from build123d import *

# Parameters (mm, degrees)
SKETCH1_R                 = 12.1666
SKETCH1_R_2               = 10.5791
BOSS_EXTRUDE1_DEPTH       = 19.05
SKETCH2_W                 = 25.4
SKETCH2_H                 = 28.575
BOSS_EXTRUDE2_DEPTH       = 3.175
SKETCH3_R                 = 6.35
CUT_EXTRUDE1_DEPTH        = 23.225
SKETCH8_R                 = 10.5791
SKETCH8_R_2               = 6.35
BOSS_EXTRUDE4_DEPTH       = 0.127
SKETCH9_R                 = 10.5791
SKETCH9_R_2               = 3.96875
BOSS_EXTRUDE5_DEPTH       = 3.175
F_2_56_TAPPED_HOLE1_D     = 1.778
F_2_56_TAPPED_HOLE1_DEPTH = 5.588
F_2_56_TAPPED_HOLE1_TIP   = 0.53416509
SKETCH6_W                 = 15.875
SKETCH6_H                 = 37.082262956
CUT_EXTRUDE2_DEPTH        = 1.5875


with BuildPart() as part:
    # Sketch1 → Boss-Extrude1 (new body)
    with BuildSketch(Plane(origin=(0, 0, 0), x_dir=(1, 0, 0), z_dir=(0, 1, 0))):
        Circle(SKETCH1_R)
        Circle(SKETCH1_R_2, mode=Mode.SUBTRACT)
    extrude(amount=BOSS_EXTRUDE1_DEPTH)

    # Sketch2 → Boss-Extrude2 (add)
    with BuildSketch(Plane.XZ):
        with Locations((0, 2.1209)):
            Rectangle(SKETCH2_W, SKETCH2_H)
    extrude(amount=BOSS_EXTRUDE2_DEPTH)

    # Sketch3 → Cut-Extrude1 (cut, through all)
    with BuildSketch(Plane.XZ.offset(3.175)):
        Circle(SKETCH3_R)
    extrude(amount=-CUT_EXTRUDE1_DEPTH, mode=Mode.SUBTRACT)

    # Sketch8 → Boss-Extrude4 (add)
    with BuildSketch(Plane(origin=(0, 0, 0), x_dir=(1, 0, 0), z_dir=(0, 1, 0))):
        Circle(SKETCH8_R)
        Circle(SKETCH8_R_2, mode=Mode.SUBTRACT)
    extrude(amount=BOSS_EXTRUDE4_DEPTH)

    # Sketch9 → Boss-Extrude5 (add)
    with BuildSketch(Plane(origin=(0, 0.127, 0), x_dir=(1, 0, 0), z_dir=(0, 1, 0))):
        Circle(SKETCH9_R)
        Circle(SKETCH9_R_2, mode=Mode.SUBTRACT)
    extrude(amount=BOSS_EXTRUDE5_DEPTH)

    # #2-56 Tapped Hole1
    with Locations(Plane(origin=(0, -3.175, 0), x_dir=(-1, 0, 0), z_dir=(0, -1, 0))):
        with Locations((10.531523735, -12.441379328), (10.531523735, 0.058620672), (-10.468476265, -12.441379328), (-10.468476265, 0.058620672)):
            Hole(F_2_56_TAPPED_HOLE1_D / 2, depth=F_2_56_TAPPED_HOLE1_DEPTH)
            with Locations((0, 0, -(F_2_56_TAPPED_HOLE1_DEPTH + F_2_56_TAPPED_HOLE1_TIP / 2))):  # 118° drill point
                Cone(0, F_2_56_TAPPED_HOLE1_D / 2, F_2_56_TAPPED_HOLE1_TIP, mode=Mode.SUBTRACT)

    # Sketch6 → Cut-Extrude2 (cut)
    with BuildSketch(Plane.XZ.offset(3.175)):
        Rectangle(SKETCH6_W, SKETCH6_H)
    extrude(amount=-CUT_EXTRUDE2_DEPTH, mode=Mode.SUBTRACT)


solid = part.part
Geometry: final body of the model. Coordinates: model frame, mm. A direction names the side the tool comes from. Coordinates: 2 decimals unless noted, no trailing zeros. Order: outer loops, then holes, each group sorted by start corner. A loop starts at its lowest first (then second) coordinate and runs counter-clockwise, first axis right, second up.
(1) Section query A-A (x = 2.5). Return the cut outline in (y, z), plus the area to 3 significant figures.
(2) Material intervals for probe 1 along X at (y, z) = (0.85, 0); probe 2 along Z at (x, y) = (0, -0.95); probe 3 along Z at (x, y) = (0, 0.9), sorted ascending.
(3) First-contact query: pin 1 (1.5 mm diameter, centred on x = 2.5, z = 1, fed in from -Y); pin 2 (10 mm diameter, centred on x = 7, y = 13.5, fed in from +Z); pin 3 (12.5 mm diameter, centred on x = 0, z = 0, fed in from -Y); pin 4 (12.5 mm diameter, centred on x = 0.5, z = -1.5, fed in from +Y). Flat tips, straight axial feed; report the tip coordinate or a pass-through.
(4) Section query B-B (y = 9.5). Return the cut outline in (x, z), plus the area to 3 significant figures.
(5) Access query for faces 5 (the face through (-7.938, -2, 2)), 6 (the face through (-11.42, -0.34, -0.1)), 7 (the face through (-4, 19.05, -10)), 8 (the face through (-7.797, 11.066, -7.15)). Directions: +Z, -Z, +X, -X, +Y, -Y. A direction counts if a zero-diameter tool reaches every point of the face in a straight line with its end or side. Return the directions, or none.
(6) Draft query along Z for faces 1 (the face through (-1.38, -0.74, 6.2)), 2 (the face through (0, -1, -12.167)), 3 (the face through (-3.6, -1.588, 5.5)), 4 (the face through (9.58, -0.34, -0.1)). Return one class per face: pulls with the +Z half, pulls with the -Z half, needs draft (parallel to the pull), parting line crosses it, or undercut.
Solution:
1. outline: (-1.59, -12.17) - (0, -12.17) - (0, -11.91) - (19.05, -11.91) - (19.05, -10.28) - (3.3, -10.28) - (3.3, -3.08) - (0.13, -3.08) - (0.13, -5.84) - (-1.59, -5.84) - close; (-1.59, 5.84) - (0.13, 5.84) - (0.13, 3.08) - (3.3, 3.08) - (3.3, 10.28) - (19.05, 10.28) - (19.05, 11.91) - (0, 11.91) - (0, 16.41) - (-1.59, 16.41) - close
1. area: 136 mm2
2. probe 1: x = -12.17 to -11.42, -9.64 to -3.97, 3.97 to 9.58, 11.36 to 12.17
2. probe 2: z = -12.17 to -6.35, 6.35 to 16.41
2. probe 3: z = -12.17 to -3.97, 3.97 to 12.17
3. pin 1: passes through
3. pin 2: stops at z = 12
3. pin 3: stops at y = 0.13
3. pin 4: stops at y = 3.3
4. outline: circle Ø24.33 at (0, 0); hole circle Ø21.16 at (0, 0)
4. area: 113 mm2
5. face 5: +Z, -Z, -Y
5. face 6: -Y
5. face 7: +Z, -Z, +X, -X, +Y
5. face 8: +Y
6. face 1: undercut
6. face 2: pulls with the -Z half
6. face 3: needs draft
6. face 4: undercut
